CAD build for the part. Positions are in the model's coordinates, mm. Face numbers are marked on the shaded views. A direction names the side the tool comes from. Give positions to 0.01 mm unless a question says otherwise; leave off trailing zeros. Order: outer loops, then holes, each group sorted by start corner. A loop starts at its lowest first (then second) coordinate and runs counter-clockwise, first axis right, second up.
```python
from build123d import *

# Parameters (mm, degrees)
SKETCH1_W           = 40
SKETCH1_H           = 40.5
BOSS_EXTRUDE1_DEPTH = 10
SKETCH2_W           = 20
SKETCH2_H           = 3.1
BOSS_EXTRUDE2_DEPTH = 7.25
SKETCH3_R           = 2.1
CUT_EXTRUDE1_DEPTH  = 43.395430178
SKETCH5_R           = 2.95
BOSS_EXTRUDE3_DEPTH = 5


with BuildPart() as part:
    # Sketch1 → Boss-Extrude1 (new, symmetric)
    with BuildSketch(Plane.YZ):
        Rectangle(SKETCH1_W, SKETCH1_H)
    extrude(amount=BOSS_EXTRUDE1_DEPTH, both=True)

    # Sketch2 → Boss-Extrude2 (add)
    with BuildSketch(Plane.XZ.offset(20)):
        with Locations((0, 9.1)):
            Rectangle(SKETCH2_W, SKETCH2_H)
    boss_extrude2 = extrude(amount=BOSS_EXTRUDE2_DEPTH)

    # Sketch3 → Cut-Extrude1 (cut, through all)
    with BuildSketch(Plane.XY.offset(10.65)):
        with Locations((-5, -24.75)):
            Circle(SKETCH3_R)
        with Locations((5, -24.75)):
            Circle(SKETCH3_R)
    cut_extrude1 = extrude(amount=-CUT_EXTRUDE1_DEPTH, mode=Mode.SUBTRACT)

    # Mirror1: Boss-Extrude2, Cut-Extrude1 across plane
    add(boss_extrude2.mirror(Plane.ZX))
    add(cut_extrude1.mirror(Plane.ZX), mode=Mode.SUBTRACT)

    # Sketch5 → Boss-Extrude3 (add)
    with BuildSketch(Plane.XY.offset(20.25)):
        with Locations((0, 10)):
            Circle(SKETCH5_R)
    extrude(amount=BOSS_EXTRUDE3_DEPTH)


solid = part.part
```
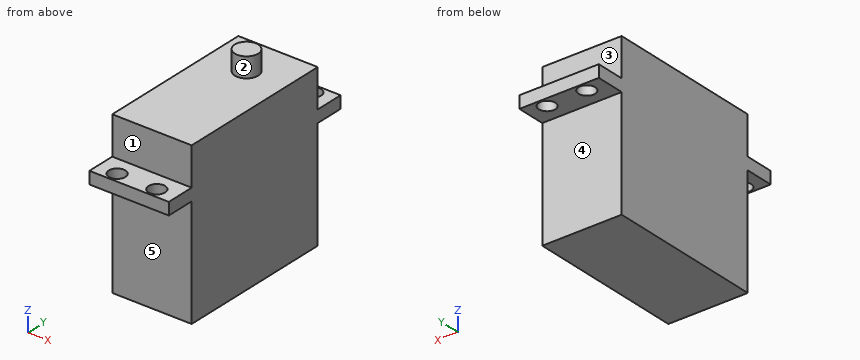
Item 1: Tool access for the marked faces 1, 2, 3, 4 and 5: list every direction of +Z, -Z, +X, -X, +Y, -Y with a clear straight run to the whole face (end or side of a thin tool).
Item 2: Drop flat-ended pins along their axis: pin 1 Ø5.5 at (x, y) = (5, -24.75) entering from +Z; pin 2 Ø2 at (x, y) = (2.5, -24.5) entering from -Z; pin 3 Ø2.5 at (x, y) = (-5, 24.75) entering from -Z; pin 4 Ø6 at (x, z) = (4, -6.5) entering from +Y. Give the stop position or say it passes through.
Item 3: Slice it at D-D (y = 10). Give the cut face in (x, z), and give its area (4 significant figures).
Item 4: Slice it at B-B (y = 24.75). Give the cut face in (x, z).
Item 5: Wall check: L1, parallel to Y at x = 5, z = 8.3; L2, parallel to Z at x = 8.75, y = 15; L3, parallel to Z at x = -7, y = -20.5. Give the ranges that are in metal, low to high.
Item 6: Slice it at C-C (x = 0). Give the cut face in (y, z).
Item 7: Slice it at A-A (x = 5). Give the cut face in (y, z).
A:
1. face 1: +Z, +X, -X, -Y
1. face 2: +Z
1. face 3: +Z, +X, -X, +Y
1. face 4: -Z, +X, -X, +Y
1. face 5: -Z, +X, -X, -Y
2. pin 1: stops at z = 10.65
2. pin 2: stops at z = 7.55
2. pin 3: passes through
2. pin 4: stops at y = 20
3. outline: (-10, -20.25) - (10, -20.25) - (10, 20.25) - (2.95, 20.25) - (2.95, 25.25) - (-2.95, 25.25) - (-2.95, 20.25) - (-10, 20.25) - close
3. area: 839.5 mm2
4. outline: (-10, 7.55) - (-7.1, 7.55) - (-7.1, 10.65) - (-10, 10.65) - close; (-2.9, 7.55) - (2.9, 7.55) - (2.9, 10.65) - (-2.9, 10.65) - close; (7.1, 7.55) - (10, 7.55) - (10, 10.65) - (7.1, 10.65) - close
5. L1: y = -27.25 to -26.85, -22.65 to 22.65, 26.85 to 27.25
5. L2: z = -20.25 to 20.25
5. L3: z = 7.55 to 10.65
6. outline: (-27.25, 7.55) - (-20, 7.55) - (-20, -20.25) - (20, -20.25) - (20, 7.55) - (27.25, 7.55) - (27.25, 10.65) - (20, 10.65) - (20, 20.25) - (12.95, 20.25) - (12.95, 25.25) - (7.05, 25.25) - (7.05, 20.25) - (-20, 20.25) - (-20, 10.65) - (-27.25, 10.65) - close
7. outline: (-27.25, 7.55) - (-26.85, 7.55) - (-26.85, 10.65) - (-27.25, 10.65) - close; (-22.65, 7.55) - (-20, 7.55) - (-20, -20.25) - (20, -20.25) - (20, 7.55) - (22.65, 7.55) - (22.65, 10.65) - (20, 10.65) - (20, 20.25) - (-20, 20.25) - (-20, 10.65) - (-22.65, 10.65) - close; (26.85, 7.55) - (27.25, 7.55) - (27.25, 10.65) - (26.85, 10.65) - close
